Build history of the part. All positions in model axes, mm. Round coordinates to 2 decimals unless told otherwise and drop trailing zeros. Loops run counter-clockwise (first coordinate to the right, second up) from the corner with the lowest first, then second, coordinate; pieces in that order, holes last. Notation, with made-up numbers: (25.25, -12) -> (38.25, -12) arc R19 ccw to (38.25, 9) -> close; hole circle Ø7 at (55, -4.5). An arc over 180 degrees is marked (long way). Put each result on its own line as item: value. Start each with the question number.
Item 1: Drill centre lines: probe 1 along X at (y, z) = (-36.5, 1.1); probe 2 along Z at (x, y) = (1.8, -17.5); probe 3 along Z at (x, y) = (1.5, -7). Where is each one in solid material? Low to high. Write a range as [from, to].
Item 2: Cut at A-A, the plane y = -28.5. List the corners of the cut face in (x, z), plus the area to 3 significant figures.
Item 3: Flat gauge pins, fed straight in: pin 1 Ø1.4 at (x, y) = (0.5, -8) entering from +Z; pin 2 Ø0.9 at (x, y) = (0.5, -22) entering from +Z. Where does each tip first touch, or does it go through?
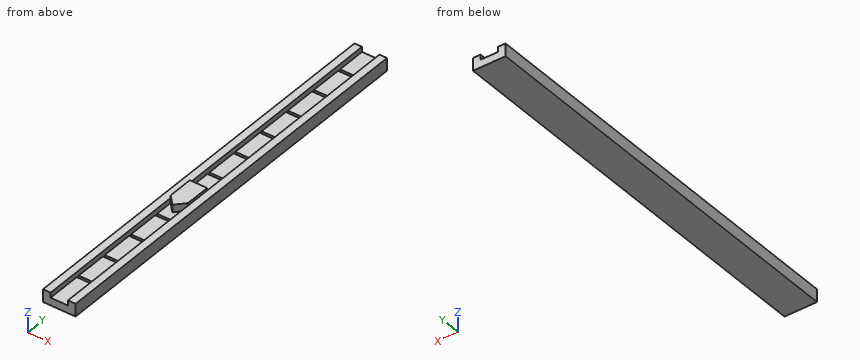
```python
from build123d import *

# Parameters (mm, degrees)
F0_W     = 1.73736
F0_H     = 41.402
F1_DEPTH = 0.762
F3_DEPTH = 0.762
F4_W     = 4.572
F4_H     = 0.254
F4_W_2   = 4.571999
F5_DEPTH = 0.508
F6_W     = 0.762
F6_H     = 41.402
F7_DEPTH = 1.27


with BuildPart() as f1:
    # F0 (on Top) → F1 (new body)
    with BuildSketch(Plane.XY):
        with Locations((0.86868, -20.5415)):
            Rectangle(F0_W, F0_H)
    extrude(amount=F1_DEPTH)

    # F2 (on face) → F3 (join)
    with BuildSketch(Plane.XY.offset(0.762)):
        Polygon((0, -22.733282), (0, -25.283881), (0.86868, -26.208002), (1.73736, -25.283881), (1.73736, -22.733282), align=None)
    extrude(amount=F3_DEPTH)

    # F4 (on face) → F5 (cut)
    with BuildSketch(Plane.XY.offset(0.762)):
        with Locations((2.078398, -37.64078)):
            Rectangle(F4_W, F4_H)
        with Locations((2.066683, -34.166079)):
            Rectangle(F4_W, F4_H)
        with Locations((2.054968, -30.691379)):
            Rectangle(F4_W, F4_H)
        with Locations((2.043252, -27.216679)):
            Rectangle(F4_W_2, F4_H)
        with Locations((2.031537, -23.741979)):
            Rectangle(F4_W, F4_H)
        with Locations((2.019822, -20.267278)):
            Rectangle(F4_W, F4_H)
        with Locations((2.008107, -16.792578)):
            Rectangle(F4_W, F4_H)
        with Locations((1.996391, -13.317878)):
            Rectangle(F4_W_2, F4_H)
        with Locations((1.984676, -9.843178)):
            Rectangle(F4_W_2, F4_H)
        with Locations((1.972961, -6.368477)):
            Rectangle(F4_W, F4_H)
        with Locations((1.961246, -2.893777)):
            Rectangle(F4_W, F4_H)
    extrude(amount=-F5_DEPTH, mode=Mode.SUBTRACT)

    # F6 (on Top) → F7 (join)
    with BuildSketch(Plane.XY):
        with Locations((-0.381, -20.5415)):
            Rectangle(F6_W, F6_H)
        with Locations((2.11836, -20.5415)):
            Rectangle(F6_W, F6_H)
    extrude(amount=F7_DEPTH)


solid = f1.part
```
Reply:
1. probe 1: x = [-0.76, 0], [1.74, 2.5]
1. probe 2: z = [0, 1.27]
1. probe 3: z = [0, 0.76]
2. outline: (-0.76, 0) -> (2.5, 0) -> (2.5, 1.27) -> (1.74, 1.27) -> (1.74, 0.76) -> (0, 0.76) -> (0, 1.27) -> (-0.76, 1.27) -> close
2. area: 3.26 mm^2
3. pin 1: stops at z = 1.27
3. pin 2: stops at z = 0.76
